from build123d import *

# Parameters (mm, degrees)
SKETCH2_W           = 180
SKETCH2_H           = 120
SKETCH2_R           = 7.5
BOSS_EXTRUDE1_DEPTH = 9.5
SKETCH14_R          = 6
SKETCH14_R_2        = 5
BOSS_EXTRUDE5_DEPTH = 18
SKETCH16_R          = 9
CUT_EXTRUDE6_DEPTH  = 156
SKETCH18_R          = 11
CUT_EXTRUDE7_DEPTH  = 156
SKETCH19_W          = 60
SKETCH19_H          = 11.842550856
CUT_EXTRUDE8_DEPTH  = 181


with BuildPart() as part:
    # Sketch2 → Boss-Extrude1 (new body, symmetric)
    with BuildSketch(Plane(origin=(0, 0, 0), x_dir=(1, 0, 0), z_dir=(0, 1, 0))):
        Rectangle(SKETCH2_W, SKETCH2_H)
        with Locations((-75, 45)):
            Circle(SKETCH2_R, mode=Mode.SUBTRACT)
        with Locations((75, 45)):
            Circle(SKETCH2_R, mode=Mode.SUBTRACT)
        with Locations((75, -45)):
            Circle(SKETCH2_R, mode=Mode.SUBTRACT)
        with Locations((-75, -45)):
            Circle(SKETCH2_R, mode=Mode.SUBTRACT)
    extrude(amount=BOSS_EXTRUDE1_DEPTH, both=True)

    # Sketch14 → Boss-Extrude5 (add, symmetric)
    with BuildSketch(Plane.XY):
        with BuildLine():
            Line((-65, 9.5), (-65, 158.5))
            ThreePointArc((-65, 158.5), (0, 223.5), (65, 158.5))
            Line((65, 158.5), (65, 9.5))
            Line((65, 9.5), (-65, 9.5))
        make_face()
        with Locations((0, 208.5)):
            Circle(SKETCH14_R, mode=Mode.SUBTRACT)
        with Locations((0, 48.5)):
            Circle(SKETCH14_R, mode=Mode.SUBTRACT)
        with Locations((-50, 158.5)):
            Circle(SKETCH14_R, mode=Mode.SUBTRACT)
        with Locations((-50, 98.5)):
            Circle(SKETCH14_R, mode=Mode.SUBTRACT)
        with Locations((50, 98.5)):
            Circle(SKETCH14_R, mode=Mode.SUBTRACT)
        with Locations((50, 158.5)):
            Circle(SKETCH14_R, mode=Mode.SUBTRACT)
        with Locations((-35.36, 63.14)):
            Circle(SKETCH14_R_2, mode=Mode.SUBTRACT)
        with Locations((35.36, 193.86)):
            Circle(SKETCH14_R_2, mode=Mode.SUBTRACT)
        with BuildLine():
            Line((-24, 133.024521594), (-24, 123.975478406))
            ThreePointArc((-24, 123.975478406), (0, 63.5), (24, 123.975478406))
            Line((24, 123.975478406), (24, 133.024521594))
            ThreePointArc((24, 133.024521594), (0, 193.5), (-24, 133.024521594))
        make_face(mode=Mode.SUBTRACT)
    extrude(amount=BOSS_EXTRUDE5_DEPTH, both=True)

    # Sketch16 → Cut-Extrude6 (cut, through all)
    with BuildSketch(Plane(origin=(65, 0, 0), x_dir=(0, 0, -1), z_dir=(1, 0, 0))):
        with Locations((0, 133.024521594)):
            Circle(SKETCH16_R)
    extrude(amount=-CUT_EXTRUDE6_DEPTH, mode=Mode.SUBTRACT)

    # Sketch18 → Cut-Extrude7 (cut, through all)
    with BuildSketch(Plane(origin=(65, 0, 0), x_dir=(0, 0, -1), z_dir=(1, 0, 0))):
        with Locations((0, 133.024521594)):
            Circle(SKETCH18_R)
    extrude(amount=-CUT_EXTRUDE7_DEPTH, mode=Mode.SUBTRACT)

    # Sketch19 → Cut-Extrude8 (cut, through all)
    with BuildSketch(Plane(origin=(90, 0, 0), x_dir=(0, 0, -1), z_dir=(1, 0, 0))):
        with Locations((0, -9.5)):
            Rectangle(SKETCH19_W, SKETCH19_H)
    extrude(amount=-CUT_EXTRUDE8_DEPTH, mode=Mode.SUBTRACT)


solid = part.part
The model under review builds one solid part; all positions refer to its coordinate system, in mm. A direction names the side the tool comes from. Coordinates: 2 decimals unless noted, no trailing zeros. Order: outer loops, then holes, each group sorted by start corner. A loop starts at its lowest first (then second) coordinate and runs counter-clockwise, first axis right, second up. Notation, with made-up numbers: (39.5, 9.5) -> (97.5, 9.5) arc R13 ccw to (97.5, 18.5) -> close; hole circle Ø1 at (31, -22.75). An arc over 180 degrees is marked (long way). Answer in a Markdown table with one row per item.
(1) The part is to be moulded in two halves that separate along X. For faces 4 (the cylindrical face through (73.37, -0.13, -37.68)), 5 (the flat face through (-1, 0, -60)), 6 (the flat face through (-90, 2, 1)), say which applies: +X half, -X half, draft (parallel to the pull), parting line (faces both ways), or undercut.
Answers:
| item | result |
|---|---|
| face 4 | undercut |
| face 5 | draft |
| face 6 | -X half |
(2) Consider section D-D (x = 75). Write out the cut boundary in (y, z).
Answers:
| item | result |
|---|---|
| outline | (-9.5, -60) -> (9.5, -60) -> (9.5, -52.5) -> (-9.5, -52.5) -> close; (-9.5, -37.5) -> (9.5, -37.5) -> (9.5, 37.5) -> (-9.5, 37.5) -> (-9.5, 30) -> (-3.58, 30) -> (-3.58, -30) -> (-9.5, -30) -> close; (-9.5, 52.5) -> (9.5, 52.5) -> (9.5, 60) -> (-9.5, 60) -> close |
(3) Consider section C-C (x = 0). Write out the cut boundary in (y, z), plus the area to 3 significant figures.
Answers:
| item | result |
|---|---|
| outline | (-9.5, -60) -> (9.5, -60) -> (9.5, -18) -> (42.5, -18) -> (42.5, 18) -> (9.5, 18) -> (9.5, 60) -> (-9.5, 60) -> (-9.5, 30) -> (-3.58, 30) -> (-3.58, -30) -> (-9.5, -30) -> close; (54.5, -18) -> (63.5, -18) -> (63.5, 18) -> (54.5, 18) -> close; (193.5, -18) -> (202.5, -18) -> (202.5, 18) -> (193.5, 18) -> close; (214.5, -18) -> (223.5, -18) -> (223.5, 18) -> (214.5, 18) -> close |
| area | 4,080 mm² |
(4) Machinability: for faces 1 (the flat face through (1, -7, 30)), 2 (the flat face through (-24, 129, 13)), 3 (the flat face through (-1, -9.5, 45)), which of the approach directions +Z, -Z, +X, -X, +Y, -Y give a long, thin tool a straight path to every point of the face, cutting with its end or side? Answer none if there is none.
Answers:
| item | result |
|---|---|
| face 1 | +X, -X, -Y |
| face 2 | +Z, -Z |
| face 3 | +Z, -Z, +X, -X, -Y |
(5) Insertion check: pin 1 (12 mm diameter, centred on y = 147.5, z = -5, fed in from -X); pin 2 (12 mm diameter, centred on x = 34, z = -11.5, fed in from +Y); pin 3 (12 mm diameter, centred on x = 31.5, z = 11, fed in from -Y); pin 4 (12 mm diameter, centred on x = -75, z = 45, fed in from +Y). Each pin has a flat end and moves straight along its axis. Give the tip position at first contact, or say it passes through.
Answers:
| item | result |
|---|---|
| pin 1 | x = -65 |
| pin 2 | y = 217.16 |
| pin 3 | y = -3.58 |
| pin 4 | through |
(6) Consider section A-A (z = 45). Write out the cut boundary in (x, y).
Answers:
| item | result |
|---|---|
| outline | (-90, -9.5) -> (-82.5, -9.5) -> (-82.5, 9.5) -> (-90, 9.5) -> close; (-67.5, -9.5) -> (67.5, -9.5) -> (67.5, 9.5) -> (-67.5, 9.5) -> close; (82.5, -9.5) -> (90, -9.5) -> (90, 9.5) -> (82.5, 9.5) -> close |
(7) Wall thickness on line 1 along Z through (x, y) = (75, -3.25); line 2 along X through (y, z) = (2.25, -45); line 3 along Y through (x, z) = (45, 0): over which ranges is each line inside the solid? List them lowest first.
Answers:
| item | result |
|---|---|
| line 1 | -60 to -52.5, -37.5 to 37.5, 52.5 to 60 |
| line 2 | -90 to -82.5, -67.5 to 67.5, 82.5 to 90 |
| line 3 | -3.58 to 95.18, 101.82 to 122.02, 144.02 to 155.18, 161.82 to 205.4 |
(8) Consider section B-B (y = 98.5). Write out the cut boundary in (x, z), plus the area to 3 significant figures.
Answers:
| item | result |
|---|---|
| outline | (-65, -18) -> (-56, -18) -> (-56, 18) -> (-65, 18) -> close; (-44, -18) -> (-35, -18) -> (-35, 18) -> (-44, 18) -> close; (35, -18) -> (44, -18) -> (44, 18) -> (35, 18) -> close; (56, -18) -> (65, -18) -> (65, 18) -> (56, 18) -> close |
| area | 1,300 mm² |
